Design review of the part built by this model. Coordinates are the model's own, in mm. A direction names the side the tool comes from. Round coordinates to 2 decimals unless told otherwise and drop trailing zeros. Order: outer loops, then holes, each group sorted by start corner. A loop starts at its lowest first (then second) coordinate and runs counter-clockwise, first axis right, second up. Notation, with made-up numbers: (43.25, 62) - (91.25, 62) arc R7 ccw to (91.25, 74) - close; hole circle Ø4 at (-16, 61). An arc over 180 degrees is marked (long way). Answer as a JSON object with one key per item and string values. Group by question number.
from build123d import *

# Parameters (mm, degrees)
SKETCH1_W           = 118
SKETCH1_H           = 142.339686002
SKETCH1_R           = 2
BOSS_EXTRUDE1_DEPTH = 4
SKETCH2_R           = 8.071067812
SKETCH2_R_2         = 7.071067812
BOSS_EXTRUDE2_DEPTH = 9
SKETCH2_4_R         = 8.071067812
SKETCH2_4_R_2       = 7.071067812
BOSS_EXTRUDE3_DEPTH = 15
CUT_EXTRUDE1_START  = -52
SKETCH2_5_R         = 7.071067812
CUT_EXTRUDE1_DEPTH  = 52
SKETCH4_R           = 1.75
SKETCH4_R_2         = 2.5
CUT_EXTRUDE2_DEPTH  = 52


with BuildPart() as part:
    # Sketch1 → Boss-Extrude1 (new body)
    with BuildSketch(Plane(origin=(0, 0, 0), x_dir=(1, 0, 0), z_dir=(0, 1, 0))):
        with Locations((6, 0)):
            Rectangle(SKETCH1_W, SKETCH1_H)
        with Locations(Location((0, 45, 0), (0, 0, 270))):
            Circle(SKETCH1_R, mode=Mode.SUBTRACT)
        with Locations(Location((60, 45, 0), (0, 0, 270))):
            Circle(SKETCH1_R, mode=Mode.SUBTRACT)
        with Locations(Location((0, 0, 0), (0, 0, 270))):
            Circle(SKETCH1_R, mode=Mode.SUBTRACT)
        with Locations(Location((60, 0, 0), (0, 0, 270))):
            Circle(SKETCH1_R, mode=Mode.SUBTRACT)
        with Locations(Location((0, -45, 0), (0, 0, 270))):
            Circle(SKETCH1_R, mode=Mode.SUBTRACT)
        with Locations(Location((60, -45, 0), (0, 0, 270))):
            Circle(SKETCH1_R, mode=Mode.SUBTRACT)
        with Locations(Location((-30, 67.5, 0), (0, 0, 270))):
            Circle(SKETCH1_R, mode=Mode.SUBTRACT)
        with Locations(Location((-30, -67.5, 0), (0, 0, 90))):
            Circle(SKETCH1_R, mode=Mode.SUBTRACT)
    extrude(amount=BOSS_EXTRUDE1_DEPTH)

    # Sketch2 → Boss-Extrude2 (add)
    # profile 1 of 3: a face of its own
    with BuildSketch(Plane(origin=(0, 4, 0), x_dir=(1, 0, 0), z_dir=(0, 1, 0))):
        with Locations(Location((-30, 43.669843001, 0), (0, 0, 270))):
            Circle(SKETCH2_R)
        with Locations(Location((-30, 43.669843001, 0), (0, 0, 270))):
            Circle(SKETCH2_R_2, mode=Mode.SUBTRACT)
    # profile 2 of 3: a face of its own
    with BuildSketch(Plane(origin=(0, 4, 0), x_dir=(1, 0, 0), z_dir=(0, 1, 0))):
        with Locations(Location((-30, -1.330156999, 0), (0, 0, 270))):
            Circle(SKETCH2_R)
        with Locations(Location((-30, -1.330156999, 0), (0, 0, 270))):
            Circle(SKETCH2_R_2, mode=Mode.SUBTRACT)
    # profile 3 of 3: a face of its own
    with BuildSketch(Plane(origin=(0, 4, 0), x_dir=(1, 0, 0), z_dir=(0, 1, 0))):
        with Locations(Location((-30, -46.330156999, 0), (0, 0, 270))):
            Circle(SKETCH2_R)
        with Locations(Location((-30, -46.330156999, 0), (0, 0, 270))):
            Circle(SKETCH2_R_2, mode=Mode.SUBTRACT)
    extrude(amount=BOSS_EXTRUDE2_DEPTH)

    # Sketch2_4 → Boss-Extrude3 (add)
    # profile 1 of 3: a face of its own
    with BuildSketch(Plane(origin=(0, 4, 0), x_dir=(1, 0, 0), z_dir=(0, 1, 0))):
        with Locations(Location((30, 43.669843001, 0), (0, 0, 270))):
            Circle(SKETCH2_4_R)
        with Locations(Location((30, 43.669843001, 0), (0, 0, 270))):
            Circle(SKETCH2_4_R_2, mode=Mode.SUBTRACT)
    # profile 2 of 3: a face of its own
    with BuildSketch(Plane(origin=(0, 4, 0), x_dir=(1, 0, 0), z_dir=(0, 1, 0))):
        with Locations(Location((30, -1.330156999, 0), (0, 0, 270))):
            Circle(SKETCH2_4_R)
        with Locations(Location((30, -1.330156999, 0), (0, 0, 270))):
            Circle(SKETCH2_4_R_2, mode=Mode.SUBTRACT)
    # profile 3 of 3: a face of its own
    with BuildSketch(Plane(origin=(0, 4, 0), x_dir=(1, 0, 0), z_dir=(0, 1, 0))):
        with Locations(Location((30, -46.330156999, 0), (0, 0, 270))):
            Circle(SKETCH2_4_R)
        with Locations(Location((30, -46.330156999, 0), (0, 0, 270))):
            Circle(SKETCH2_4_R_2, mode=Mode.SUBTRACT)
    extrude(amount=BOSS_EXTRUDE3_DEPTH)

    # Sketch2_5 → Cut-Extrude1 (cut)
    with BuildSketch(Plane(origin=(0, 4, 0), x_dir=(1, 0, 0), z_dir=(0, 1, 0)).offset(CUT_EXTRUDE1_START)):
        with Locations(Location((30, -46.330156999, 0), (0, 0, 270))):
            Circle(SKETCH2_5_R)
        with Locations(Location((-30, -46.330156999, 0), (0, 0, 270))):
            Circle(SKETCH2_5_R)
        with Locations(Location((-30, -1.330156999, 0), (0, 0, 270))):
            Circle(SKETCH2_5_R)
        with Locations(Location((-30, 43.669843001, 0), (0, 0, 270))):
            Circle(SKETCH2_5_R)
        with Locations(Location((30, 43.669843001, 0), (0, 0, 270))):
            Circle(SKETCH2_5_R)
        with Locations(Location((30, -1.330156999, 0), (0, 0, 270))):
            Circle(SKETCH2_5_R)
    extrude(amount=CUT_EXTRUDE1_DEPTH, mode=Mode.SUBTRACT)

    # Sketch4 → Cut-Extrude2 (cut)
    with BuildSketch(Plane.XZ):
        with Locations(Location((40, -21.169843001, 0), (0, 0, 270))):
            Circle(SKETCH4_R)
        with Locations(Location((20, -21.169843001, 0), (0, 0, 270))):
            Circle(SKETCH4_R)
        with Locations(Location((30, -21.169843001, 0), (0, 0, 270))):
            Circle(SKETCH4_R_2)
        with Locations(Location((-40, -21.169843001, 0), (0, 0, 270))):
            Circle(SKETCH4_R)
        with Locations(Location((-30, -21.169843001, 0), (0, 0, 270))):
            Circle(SKETCH4_R_2)
        with Locations(Location((-20, -21.169843001, 0), (0, 0, 270))):
            Circle(SKETCH4_R)
        with Locations(Location((-40, 23.830156999, 0), (0, 0, 270))):
            Circle(SKETCH4_R)
        with Locations(Location((-30, 23.830156999, 0), (0, 0, 270))):
            Circle(SKETCH4_R_2)
        with Locations(Location((-20, 23.830156999, 0), (0, 0, 270))):
            Circle(SKETCH4_R)
        with Locations(Location((20, 23.830156999, 0), (0, 0, 270))):
            Circle(SKETCH4_R)
        with Locations(Location((30, 23.830156999, 0), (0, 0, 270))):
            Circle(SKETCH4_R_2)
        with Locations(Location((40, 23.830156999, 0), (0, 0, 270))):
            Circle(SKETCH4_R)
    extrude(amount=-CUT_EXTRUDE2_DEPTH, mode=Mode.SUBTRACT)


solid = part.part
1. To check wall thickness, follow line 1 (Z direction, x = -32.5, y = 7.25); line 2 (Z direction, x = 59, y = 3); line 3 (Y direction, x = 16, z = -29.5). State the ranges of each line that lie inside material, in increasing order. Write a range as from..to.
2. Take a section at C-C, the plane z = -67.5. Give the boundary of the cut face in (x, y).
3. Take a section at D-D, the plane y = 9. Count the separate pieces of the cut face and the enclosed holes in it, then the cut area to 3 significant figures.
4. Clearance check with flat-ended pins moving along their axes: P1, Ø6.5, axis at x = 60, z = -45, coming from the +Y side; P2, Ø2, axis at x = 32.5, y = 6.5, coming from the +Z side; P3, Ø18, axis at x = -27, z = -40.5, coming from the +Y side; P4, Ø3, axis at x = 20, z = -21.17, coming from the +Y side. State where each tip first meets the part, or that it passes through.
5. Take a section at A-A, the plane x = -20. Give the boundary of the cut face in (y, z), then the cut area to 3 significant figures.
6. Mouldability with a two-part tool opening along Z and no side actions: class faces 3 (the cylindrical face through (62, 2, -45)), 4 (the cylindrical face through (32.11, 1.97, 22.49)), 5 (the flat face through (23, 19, -41)) as pulls with the +Z half, pulls with the -Z half, needs draft (parallel to the pull), parting line crosses it, or undercut.
7. Take a section at B-B, the plane y = 16.75. Give the boundary of the cut face in (x, z).
8. Tool access review of faces 1 (the cylindrical face through (32.11, 1.97, -22.51)), 2 (the flat face through (-37, 13, -41)): name each direction out of +Z, -Z, +X, -X, +Y, -Y from which nothing blocks a thin tool from reaching the whole face with its end or side.
Response values:
{
 "1": {"line 1": "-51.34..-50.28, -37.06..-36, -6.34..-5.28, 7.94..9, 38.66..39.72, 52.94..54", "line 2": "-71.17..-46.73, -43.27..-1.73, 1.73..43.27, 46.73..71.17", "line 3": "0..4"},
 "2": {"outline": "(-53, 0) - (-32, 0) - (-32, 4) - (-53, 4) - close; (-28, 0) - (65, 0) - (65, 4) - (-28, 4) - close"},
 "3": {"separate pieces": "6", "enclosed holes": "6", "area": "285 mm2"},
 "4": {"P1": "y = 4", "P2": "z = 54.26", "P3": "y = 13", "P4": "through"},
 "5": {"outline": "(0, -71.17) - (4, -71.17) - (4, -22.92) - (0, -22.92) - close; (0, -19.42) - (4, -19.42) - (4, 22.08) - (0, 22.08) - close; (0, 25.58) - (4, 25.58) - (4, 71.17) - (0, 71.17) - close", "area": "541 mm2"},
 "6": {"face 3": "undercut", "face 4": "undercut", "face 5": "needs draft"},
 "7": {"outline": "circle Ø16.14 at (30, -43.67); circle Ø16.14 at (30, 1.33); circle Ø16.14 at (30, 46.33); hole circle Ø14.14 at (30, -43.67); hole circle Ø14.14 at (30, 1.33); hole circle Ø14.14 at (30, 46.33)"},
 "8": {"face 1": "+Y, -Y", "face 2": "+Z, -Z, -X, +Y"}
}
